```python
from build123d import *

# Parameters (mm, degrees)
SKETCH1_R           = 6.35
BOSS_EXTRUDE1_DEPTH = 7.9375
SKETCH2_R           = 2.2
CUT_EXTRUDE1_DEPTH  = 12.985362166
SKETCH3_R           = 1
CUT_EXTRUDE2_DEPTH  = 3.4


with BuildPart() as part:
    # Sketch1 → Boss-Extrude1 (new body)
    with BuildSketch(Plane(origin=(0, 0, 0), x_dir=(1, 0, 0), z_dir=(0, 1, 0))):
        with Locations(Location((0, 0, 0), (0, 0, 270))):
            Circle(SKETCH1_R)
    extrude(amount=BOSS_EXTRUDE1_DEPTH)

    # Sketch2 → Cut-Extrude1 (cut, through all)
    with BuildSketch(Plane.XZ):
        with Locations(Location((-3.49, 0, 0), (0, 0, 270))):
            Circle(SKETCH2_R)
    extrude(amount=-CUT_EXTRUDE1_DEPTH, mode=Mode.SUBTRACT)

    # Sketch3 → Cut-Extrude2 (cut)
    with BuildSketch(Plane.XZ):
        with Locations(Location((-3.49, -3.8, 0), (0, 0, 270))):
            Circle(SKETCH3_R)
        with Locations(Location((-3.49, 3.8, 0), (0, 0, 270))):
            Circle(SKETCH3_R)
    extrude(amount=-CUT_EXTRUDE2_DEPTH, mode=Mode.SUBTRACT)


solid = part.part
```
Geometry: final body of the model. Coordinates: model frame, mm. A direction names the side the tool comes from. Give positions to 0.01 mm unless a question says otherwise; leave off trailing zeros. Loops run counter-clockwise (first coordinate to the right, second up) from the corner with the lowest first, then second, coordinate; pieces in that order, holes last. Notation, with made-up numbers: (-12, 72) -> (-6, 72) arc R22 cw to (-6, 103) -> close; hole circle Ø6 at (-21, -16.75). An arc over 180 degrees is marked (long way). Use one line per item in the form item = value.
Item 1: Draft query along X for faces 1 (the face through (0, 0, 0)), 2 (the face through (-3, 3.4, 4)), 3 (the face through (-3.86, 3.91, -5.04)). Return one class per face: pulls with the +X half, pulls with the -X half, needs draft (parallel to the pull), parting line crosses it, or undercut.
A:
face_1 = needs draft
face_2 = undercut
face_3 = parting line crosses it
Item 2: Section query A-A on z = 0. Output: boundary loops of the cut face in (x, y), and give its area (3 significant figures).
A:
outline = (-6.35, 0) -> (-5.69, 0) -> (-5.69, 7.94) -> (-6.35, 7.94) -> close; (-1.29, 0) -> (6.35, 0) -> (6.35, 7.94) -> (-1.29, 7.94) -> close
area = 65.9 mm^2
Item 3: Section query D-D on y = 5. Output: boundary loops of the cut face in (x, z).
A:
outline = circle Ø12.7 at (0, 0); hole circle Ø4.4 at (-3.49, 0)
Item 4: Section query C-C on y = 0.5. Output: boundary loops of the cut face in (x, z).
A:
outline = circle Ø12.7 at (0, 0); hole circle Ø4.4 at (-3.49, 0); hole circle Ø2 at (-3.49, -3.8); hole circle Ø2 at (-3.49, 3.8)
Item 5: Section query B-B on x = -3.49. Output: boundary loops of the cut face in (y, z).
A:
outline = (0, -5.3) -> (7.94, -5.3) -> (7.94, -2.2) -> (0, -2.2) -> (0, -2.8) -> (3.4, -2.8) -> (3.4, -4.8) -> (0, -4.8) -> close; (0, 2.2) -> (7.94, 2.2) -> (7.94, 5.3) -> (0, 5.3) -> (0, 4.8) -> (3.4, 4.8) -> (3.4, 2.8) -> (0, 2.8) -> close
Item 6: Line query: probe 1 along Z at (x, y) = (-3, 0.75); probe 2 along X at (y, z) = (4.25, 0); probe 3 along X at (y, z) = (2, 0.75). Output: solid intervals per line, ascending.
A:
probe_1 = -5.6 to -4.67, -2.93 to -2.14, 2.14 to 2.93, 4.67 to 5.6
probe_2 = -6.35 to -5.69, -1.29 to 6.35
probe_3 = -6.31 to -5.56, -1.42 to 6.31
Item 7: Pin query (flat end, axial travel): P1, Ø2, axis at x = 3.5, y = 4, coming from the -Z side. Return the tip coordinate at first contact, or that it passes through.
A:
P1 = -5.84
Item 8: Access query for faces 4 (the face through (-2.814, 1.676, -3.063)), 5 (the face through (-5.638, 3.913, 0.477)). Directions: +Z, -Z, +X, -X, +Y, -Y. A direction counts if a zero-diameter tool reaches every point of the face in a straight line with its end or side. Return the directions, or none.
A:
face_4 = -Y
face_5 = +Y, -Y
